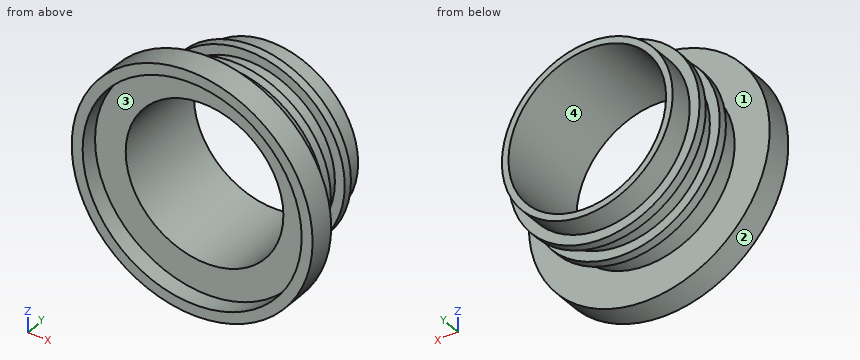
from build123d import *

# Parameters (mm, degrees)
SKETCH_1_R          = 19.5
SKETCH_1_R_2        = 18
EXTRUDE_1_DEPTH     = 20
SKETCH_3_R          = 27.5
EXTRUDE_2_DEPTH     = 2
SKETCH_4_R          = 21.75
EXTRUDE_3_DEPTH     = 2
EXTRUDE_START       = 1
SKETCH_8_R          = 21.75
EXTRUDE_4_DEPTH     = 2
SKETCH_6_R          = 18
CUT_EXTRUDE_1_DEPTH = 35
SKETCH_13_R         = 27.5
SKETCH_13_R_2       = 25
EXTRUDE_6_DEPTH     = 4
SKETCH_13_4_R       = 18
CUT_EXTRUDE_2_DEPTH = 23.5


with BuildPart() as part:
    # Sketch 1 → Extrude 1 (new body)
    with BuildSketch(Plane(origin=(0, 0, 0), x_dir=(1, 0, 0), z_dir=(0, 1, 0))):
        Circle(SKETCH_1_R)
        Circle(SKETCH_1_R_2, mode=Mode.SUBTRACT)
    extrude(amount=EXTRUDE_1_DEPTH)

    # Sketch 3 → Extrude 2 (add)
    with BuildSketch(Plane.XZ):
        Circle(SKETCH_3_R)
    extrude(amount=EXTRUDE_2_DEPTH)

    # Sketch 4 → Extrude 3 (add)
    with BuildSketch(Plane(origin=(0, 8, 0), x_dir=(1, 0, 0), z_dir=(0, 1, 0))):
        Circle(SKETCH_4_R)
    extrude(amount=-EXTRUDE_3_DEPTH)

    # Sketch 8 → Extrude 4 (add)
    with BuildSketch(Plane(origin=(0, 11.5, 0), x_dir=(1, 0, 0), z_dir=(0, 1, 0)).offset(EXTRUDE_START)):
        Circle(SKETCH_8_R)
    extrude(amount=EXTRUDE_4_DEPTH)

    # Sketch 6 → Cut-Extrude 1 (cut)
    with BuildSketch(Plane(origin=(0, 0, 0), x_dir=(1, 0, 0), z_dir=(0, 1, 0))):
        Circle(SKETCH_6_R)
    extrude(amount=CUT_EXTRUDE_1_DEPTH, mode=Mode.SUBTRACT)

    # Sketch 13 → Extrude 6 (add)
    with BuildSketch(Plane.XZ.offset(2)):
        Circle(SKETCH_13_R)
        Circle(SKETCH_13_R_2, mode=Mode.SUBTRACT)
    extrude(amount=EXTRUDE_6_DEPTH)

    # Sketch 13_4 → Cut-Extrude 2 (cut)
    with BuildSketch(Plane.XZ.offset(2)):
        Circle(SKETCH_13_4_R)
    extrude(amount=-CUT_EXTRUDE_2_DEPTH, mode=Mode.SUBTRACT)


solid = part.part
Read the model definition and answer for the solid it produces. Units are mm, in the model's axes. Face numbers are marked on the shaded views. Give positions to 0.01 mm unless a question says otherwise; leave off trailing zeros. Write each loop counter-clockwise with the first axis right and the second up, starting at its lowest first coordinate (ties: lowest second). Pieces come first, ordered by that corner, then holes. Notation, with made-up numbers: M -20.5,85 L 17.5,85 A16 ccw 17.5,101 Z; hole C -15,-13 d6. An arc over 180 degrees is marked long. One line per item, written item: value. Start each with the question number.
(1) Find section C-C (y = 7). Determine the outline of the cut face in (x, z).
(2) Find the intervals of material crossed by line 1 (Y direction, x = -5, z = 20.5); line 2 (Z direction, x = 0, y = 15.5); line 3 (Z direction, x = 0, y = -4.55), in increasing order.
(3) Flat-ended cylindrical pins translate along their axes: pin 1 Ø4 at (x, y) = (-16.5, 5) entering from +Z; pin 2 Ø1.5 at (y, z) = (11, -0.5) entering from +X; pin 3 Ø10 at (x, y) = (0.5, 3) entering from +Z. Find the tip coordinate at first contact, or state that the pin passes through.
(4) Find section D-D (z = 24). Determine the outline of the cut face in (x, y), plus the area to 3 significant figures.
(5) Determine the mould class of the marked faces 1, 2, 3 and 4 for opening direction Z: pulls with the +Z half, pulls with the -Z half, needs draft (parallel to the pull), parting line crosses it, or undercut.
Results below:
1. outline: C 0,0 d43.5; hole C 0,0 d36
2. line 1: y = -2 to 0, 6 to 8, 12.5 to 14.5
2. line 2: z = -19.5 to -18, 18 to 19.5
2. line 3: z = -27.5 to -25, 25 to 27.5
3. pin 1: stops at z = 15.97
3. pin 2: stops at x = 19.5
3. pin 3: stops at z = 27.5
4. outline: M -13.43,-6 L -7,-6 L -7,-2 L 7,-2 L 7,-6 L 13.43,-6 L 13.43,0 L -13.43,0 Z
4. area: 105 mm^2
5. face 1: needs draft
5. face 2: parting line crosses it
5. face 3: undercut
5. face 4: undercut
